Check sheet for the modelled part. Datum: model origin and axes. Units: mm. Face numbers are marked on the shaded views. Round coordinates to 2 decimals unless told otherwise and drop trailing zeros. Loops run counter-clockwise (first coordinate to the right, second up) from the corner with the lowest first, then second, coordinate; pieces in that order, holes last. Notation, with made-up numbers: (-28, 56.25) -> (-24, 56.25) arc R19 cw to (-24, 92.25) -> close; hole circle Ø3 at (38, 76.25). An arc over 180 degrees is marked (long way). Use one line per item in the form item = value. Start each with the question number.
(1) Sectioned sample at B-B (x = 110). Record the cut outline in (y, z).
(2) Sectioned sample at D-D (y = 18.5). Record the cut outline in (x, z), and give its area (3 significant figures).
(3) Material ranges on probe 1 along X at (y, z) = (46, 2.25); probe 2 along X at (y, z) = (36.5, 3.75); probe 3 along Z at (x, y) = (17.5, 17), recorded low to high. Write a range as [from, to].
(4) Sectioned sample at A-A (y = 40.5). Record the cut outline in (x, z), and give its area (3 significant figures).
(5) Go/stop test with a flat-tipped pin: pin 1 (3 mm diameter, centred on x = 87.5, y = 14.5, fed in from -Z). Record where the tip stops, or that it passes through.
(6) Sectioned sample at C-C (z = 4). Record the cut outline in (x, y).
(7) Draft check along X on the marked faces 1, 2 and 3. Enter one of: released by +X, released by -X, zero draft, split by the parting line, or undercut.
from build123d import *

# Parameters (mm, degrees)
RESSALTO_EXTRUS_O1_DEPTH = 8
CORTE_EXTRUS_O1_DEPTH    = 134.940285202


with BuildPart() as part:
    # Esboço1 → Ressalto-extrusão1 (new body)
    with BuildSketch(Plane.XY):
        Polygon((0, 0), (124, 0), (124, 50), (94, 35), (30, 35), (0, 50), align=None)
    extrude(amount=RESSALTO_EXTRUS_O1_DEPTH)

    # Esboço2 → Corte-extrusão1 (cut, through all)
    with BuildSketch(Plane.ZY):
        Polygon((8, 0), (0, 0), (0, 19.800694827), align=None)
    extrude(amount=-CORTE_EXTRUS_O1_DEPTH, mode=Mode.SUBTRACT)


solid = part.part
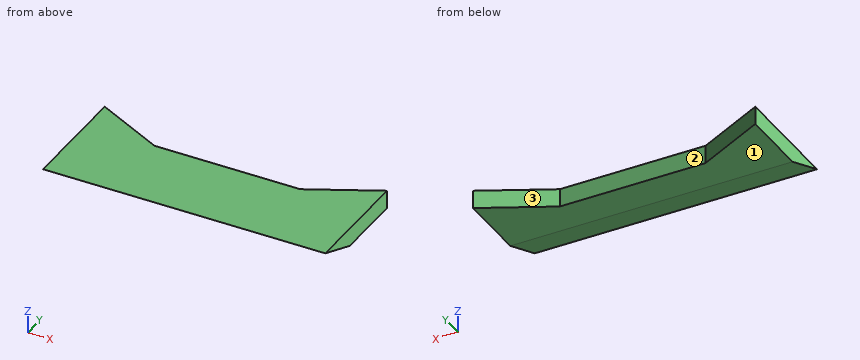
Checks:
q1.outline = (0, 8) -> (19.8, 0) -> (43, 0) -> (43, 8) -> close
q2.outline = (0, 0.53) -> (124, 0.53) -> (124, 8) -> (0, 8) -> close
q2.area = 927 mm2
q3.probe_1 = [0, 8], [116, 124]
q3.probe_2 = [0, 27], [97, 124]
q3.probe_3 = [1.13, 8]
q4.outline = (0, 0) -> (19, 0) -> (19, 8) -> (0, 8) -> close; (105, 0) -> (124, 0) -> (124, 8) -> (105, 8) -> close
q4.area = 304 mm2
q5.pin_1 = 1.54
q6.outline = (0, 9.9) -> (124, 9.9) -> (124, 50) -> (94, 35) -> (30, 35) -> (0, 50) -> close
q7.face_1 = zero draft
q7.face_2 = undercut
q7.face_3 = undercut
